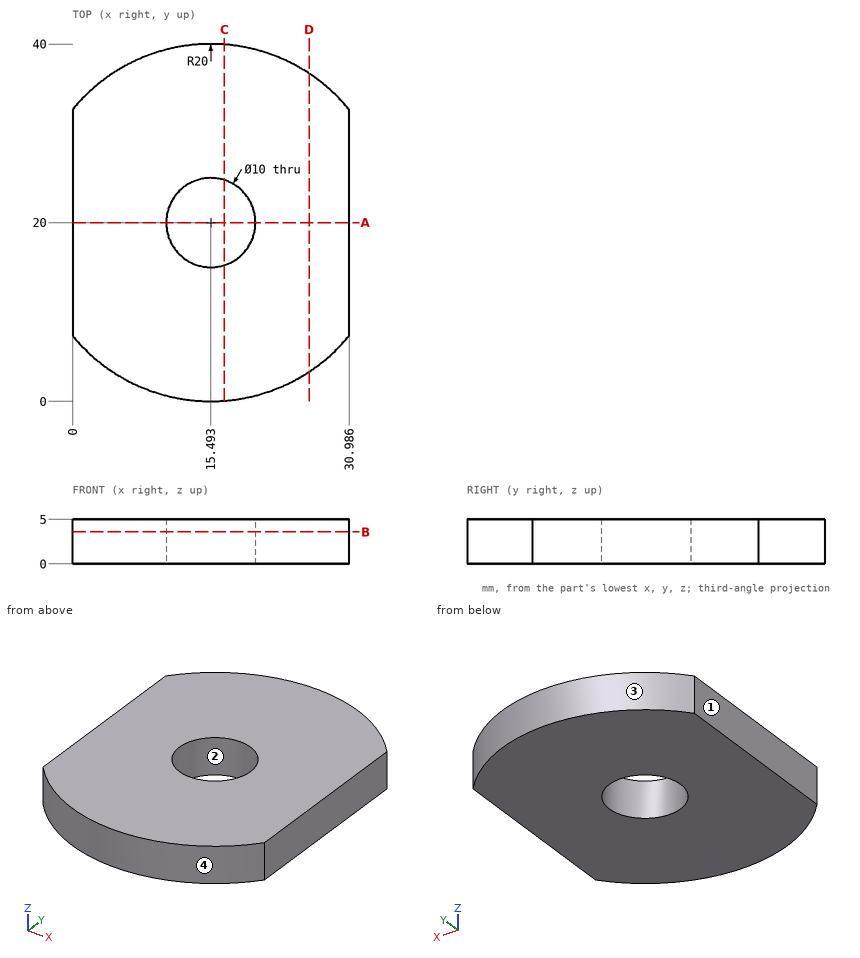
Design review of the part shown in the three views and the two pictorial views. Dimensions are in mm from the part's minimum x, y and z. Coordinates: 2 decimals unless noted, no trailing zeros. Loops run counter-clockwise (first coordinate to the right, second up) from the corner with the lowest first, then second, coordinate; pieces in that order, holes last.
(1) Consider section B-B, the plane z = 3.6. Give the boundary of the cut face in (x, y) (1 decimal).
Determined:
outline: (0, 7.4) arc R20 ccw to (31, 7.4) - (31, 32.6) arc R20 ccw to (0, 32.6) - close; hole circle Ø10 at (15.5, 20)
(2) Wall thickness on L1, parallel to X at y = 18, z = 4.25 (1 decimal); L2, parallel to Y at x = 14.5, z = 2.8 (1 decimal); L3, parallel to Y at x = 3, z = 4.5: over which ranges is each line inside the solid? List them lowest first.
Determined:
L1: x = 0 to 10.9, 20.1 to 31
L2: y = 0 to 15.1, 24.9 to 40
L3: y = 4.38 to 35.62
(3) Consider section C-C, the plane x = 17. Give the boundary of the cut face in (y, z).
Determined:
outline: (0.06, 0) - (15.23, 0) - (15.23, 5) - (0.06, 5) - close; (24.77, 0) - (39.94, 0) - (39.94, 5) - (24.77, 5) - close
(4) Consider section D-D, the plane x = 26.5. Give the boundary of the cut face in (y, z), plus the area to 3 significant figures.
Determined:
outline: (3.3, 0) - (36.7, 0) - (36.7, 5) - (3.3, 5) - close
area: 167 mm2
(5) Insertion check: P1, Ø2, axis at x = 24.5, z = 1, coming from the +Y side. The pin has a flat end and moves straight along its axis. Give the tip position at first contact, or say it passes through.
Determined:
P1: stops at y = 38.33
(6) Consider section A-A, the plane y = 20. Give the boundary of the cut face in (x, z) (1 decimal).
Determined:
outline: (0, 0) - (10.5, 0) - (10.5, 5) - (0, 5) - close; (20.5, 0) - (31, 0) - (31, 5) - (20.5, 5) - close
(7) Draft analysis for pull direction Y (two halves, no side actions). For the marked faces 1, 2, 3 and 4, state which applies: +Y half, -Y half, draft (parallel to the pull), parting line (faces both ways), or undercut.
Determined:
face 1: draft
face 2: undercut
face 3: +Y half
face 4: -Y half
